Model file for the job. Use its own axes, mm. A direction names the side the tool comes from. Coordinates: 2 decimals unless noted, no trailing zeros. Order: outer loops, then holes, each group sorted by start corner. A loop starts at its lowest first (then second) coordinate and runs counter-clockwise, first axis right, second up.
Autodesk Inventor part; units mm, degrees
ref_plane "YZ Plane" through (0, 0, 0) normal (1, 0, 0) x (0, 1, 0)
ref_plane "XZ Plane" through (0, 0, 0) normal (0, 1, 0) x (-1, 0, 0)
ref_plane "XY Plane" through (0, 0, 0) normal (0, 0, 1) x (1, 0, 0)
sketch "Sketch1" plane through (0, 0, 0) normal (0, 0, 1) x (1, 0, 0)
  circle A0 centre (0, -31) radius 1.6
  circle A1 centre (0, 0) radius 13.5
  circle A2 centre (0, 0) radius 20
  line L0 (0, 0) -> (0, -31) construction
  line L1 (0, -31) -> (0, -7.0396) construction
  line L2 (-3.1, -31) -> (-3.1, -19.7583)
  arc A3 (-3.1, -31) -> (3.1, -31) centre (0, -31) ccw
  line L3 (3.1, -19.7583) -> (3.1, -31)
  circle A4 centre (26.8468, 15.5) radius 1.6
  line L4 (0, 0) -> (26.8468, 15.5) construction
  line L5 (26.8468, 15.5) -> (6.0965, 3.5198) construction
  line L6 (28.3968, 12.8153) -> (18.6612, 7.1945)
  arc A5 (28.3968, 12.8153) -> (25.2968, 18.1847) centre (26.8468, 15.5) ccw
  line L7 (15.5612, 12.5638) -> (25.2968, 18.1847)
  circle A6 centre (-26.8468, 15.5) radius 1.6
  line L8 (0, 0) -> (-26.8468, 15.5) construction
  line L9 (-26.8468, 15.5) -> (-6.0965, 3.5198) construction
  line L10 (-25.2968, 18.1847) -> (-15.5612, 12.5638)
  arc A7 (-25.2968, 18.1847) -> (-28.3968, 12.8153) centre (-26.8468, 15.5) ccw
  line L11 (-18.6612, 7.1945) -> (-28.3968, 12.8153)
  point P0 (18.6612, 7.1945)
  point P1 (15.5612, 12.5638)
  dimension "d4" = 31
  dimension "d5" = 3.2
  dimension "d6" = 27
  dimension "d7" = 40
  dimension "d8" = 1.5
  dimension "d11" = 360
extrude "Extrusion1" add sketch "Sketch1" along normal blind 1.5
fillet "Fillet1" radius 5 6 edges at (-15.5612, 12.5638, 0.75) (15.5612, 12.5638, 0.75) (18.6612, 7.1945, 0.75) (-18.6612, 7.1945, 0.75) (-3.1, -19.7583, 0.75) (3.1, -19.7583, 0.75)
sketch "Sketch2" plane through (0, 0, 1.5) normal (0, 0, 1) x (1, 0, 0)
  arc A0 (-20.2121, 10.7235) -> (-0.8192, -22.866) centre (-6.2805, -3.626) ccw construction
  arc A1 (0.8192, -22.866) -> (20.2121, 10.7235) centre (6.2805, -3.626) ccw construction
  circle A2 centre (0, 0) radius 13.5 construction
  arc A3 (-20.3166, 10.8312) -> (-0.75, -23.0022) centre (-6.2805, -3.626) ccw
  arc A4 (0.75, -23.0022) -> (19.7139, 11.3928) centre (6.2805, -3.626) ccw
  line L0 (-0.75, -23.0022) -> (0.75, -23.0022)
  line L1 (25.2968, 18.1847) -> (18.9327, 14.5104)
  arc A5 (13.1462, 15.0724) -> (18.9327, 14.5104) centre (16.4327, 18.8405) ccw
  arc A6 (13.1462, 15.0724) -> (-13.1462, 15.0724) centre (0, 0) ccw
  arc A7 (-18.9327, 14.5104) -> (-13.1462, 15.0724) centre (-16.4327, 18.8405) ccw
  line L2 (-18.9327, 14.5104) -> (-25.2968, 18.1847)
  arc A8 (-25.2968, 18.1847) -> (-28.3968, 12.8153) centre (-26.8468, 15.5) ccw
  line L3 (-28.3968, 12.8153) -> (-22.0327, 9.141)
  arc A9 (-19.6262, 3.8487) -> (-22.0327, 9.141) centre (-24.5327, 4.8109) ccw
  arc A10 (-19.6262, 3.8487) -> (-6.48, -18.9211) centre (0, 0) ccw
  arc A11 (-3.1, -23.6514) -> (-6.48, -18.9211) centre (-8.1, -23.6514) ccw
  line L4 (-3.1, -23.6514) -> (-3.1, -31)
  arc A12 (-3.1, -31) -> (3.1, -31) centre (0, -31) ccw
  line L5 (3.1, -31) -> (3.1, -23.6514)
  arc A13 (6.48, -18.9211) -> (3.1, -23.6514) centre (8.1, -23.6514) ccw
  arc A14 (6.48, -18.9211) -> (19.6262, 3.8487) centre (0, 0) ccw
  arc A15 (22.0327, 9.141) -> (19.6262, 3.8487) centre (24.5327, 4.8109) ccw
  line L6 (22.0327, 9.141) -> (28.3968, 12.8153)
  arc A16 (28.3968, 12.8153) -> (25.2968, 18.1847) centre (26.8468, 15.5) ccw
  circle A17 centre (0, -31) radius 1.6
  circle A18 centre (0, 0) radius 13.5
  circle A19 centre (26.8468, 15.5) radius 1.6
  circle A20 centre (-26.8468, 15.5) radius 1.6
  arc A21 (19.5455, 12.1506) -> (-19.7234, 11.3763) centre (0, 7.2521) ccw
  arc A22 (0.7782, -23.0103) -> (20.2955, 10.8516) centre (6.2805, -3.626) ccw
  line L7 (20.2955, 10.8516) -> (19.5455, 12.1506)
  arc A23 (-20.2955, 10.8516) -> (0.0095, -22.7691) centre (-6.2805, -3.626) ccw
  arc A24 (19.5383, 12.1791) -> (-19.5455, 12.1506) centre (0, 7.2521) ccw
  line L8 (-19.5455, 12.1506) -> (-20.2955, 10.8516)
  point P0 (3.1016, -23.5237)
  point P1 (-3.1016, -23.5237)
  point P2 (18.8213, 14.4479)
  point P3 (20.2955, 10.8516)
  point P4 (21.9229, 9.0758)
  point P5 (-21.9229, 9.0758)
  point P6 (-20.3166, 10.8312)
  point P7 (-19.5455, 12.1506)
  point P8 (-18.8213, 14.4479)
  dimension "d16" = 0.15
  dimension "d17" = 0.15
  dimension "d18" = 1.5
  dimension "d21" = 360
extrude "Extrusion2" add sketch "Sketch2" along normal blind 3 contours A3 A9 L3 A8 L2 A7 A21 L8 A23 | A3 L0 A4 A13 L5 A12 L4 A11 | A5 L1 A16 L6 A15 A4 L7 A21
properties part number "Bracket"
Q1. Drop flat-ended pins along their axis: P1, Ø3, axis at x = 25, y = 11, coming from the -Z side; P2, Ø1.5, axis at y = -20.5, z = 1.5, coming from the -X side. Give the stop position or say it passes through.
Established:
P1: stops at z = 0
P2: stops at x = -4.97
Q2. Probe line 1 (Y direction, x = 0, z = 0.6); line 2 (Y direction, x = 0, z = 3.05); line 3 (Z direction, x = -12.5, y = -9). List the from-to ranges inside material, lowest first.
Established:
line 1: y = -34.1 to -32.6, -29.4 to -13.5, 13.5 to 20
line 2: y = -34.1 to -32.6, -29.4 to -23
line 3: z = 0 to 1.5
Q3. Cut at D-D, the plane x = 9.5. List the corners of the cut face in (y, z), plus the area to 3 significant figures.
Established:
outline: (-17.6, 0) - (-9.59, 0) - (-9.59, 1.5) - (-17.6, 1.5) - close; (9.59, 0) - (17.6, 0) - (17.6, 1.5) - (9.59, 1.5) - close
area: 24.0 mm2
Q4. Cut at A-A, the plane y = 0. List the corners of the cut face in (x, z).
Established:
outline: (-20, 0) - (-13.5, 0) - (-13.5, 1.5) - (-20, 1.5) - close; (13.5, 0) - (20, 0) - (20, 1.5) - (13.5, 1.5) - close
Q5. Cut at C-C, the plane x = 0. List the corners of the cut face in (y, z).
Established:
outline: (-34.1, 0) - (-32.6, 0) - (-32.6, 4.5) - (-34.1, 4.5) - close; (-29.4, 0) - (-13.5, 0) - (-13.5, 1.5) - (-23, 1.5) - (-23, 4.5) - (-29.4, 4.5) - close; (13.5, 0) - (20, 0) - (20, 1.5) - (13.5, 1.5) - close
Q6. Which spindle directions (+Z, -Z, +X, -X, +Y, -Y) get a long thin tool onto all of the face, cutting with end or side? Do faces 5 (the face through (-24, 14, 4.5)), 6 (the face through (-19.963, 6.841, 0.76)), 7 (the face through (0, -23.002, 3)), 8 (the face through (19.926, 11.492, 2.979)), 9 (the face through (-22.159, 16.373, 0.74)). Say none if no direction does.
Established:
face 5: +Z, +X, -X, +Y, -Y
face 6: +Z, -Z, -X
face 7: +Z, +X, -X, +Y
face 8: +Z, -Y
face 9: +Z, -Z, +Y
Q7. Cut at B-B, the plane z = 2.25. Count the separate pieces of the cut face and the enclosed holes in it, plus the area to 3 significant figures.
Established:
separate pieces: 3
enclosed holes: 3
area: 166 mm2
Q8. Mould opens along X. For faces 1 (the face through (3.1, -27, 2)), 2 (the face through (19.21, 13.33, 2.98)), 3 (the face through (22.159, 16.373, 2.979)), 4 (the face through (24, 14, 4.5)) say: pulls with the +X half, pulls with the -X half, needs draft (parallel to the pull), parting line crosses it, or undercut.
Established:
face 1: pulls with the +X half
face 2: undercut
face 3: undercut
face 4: needs draft
